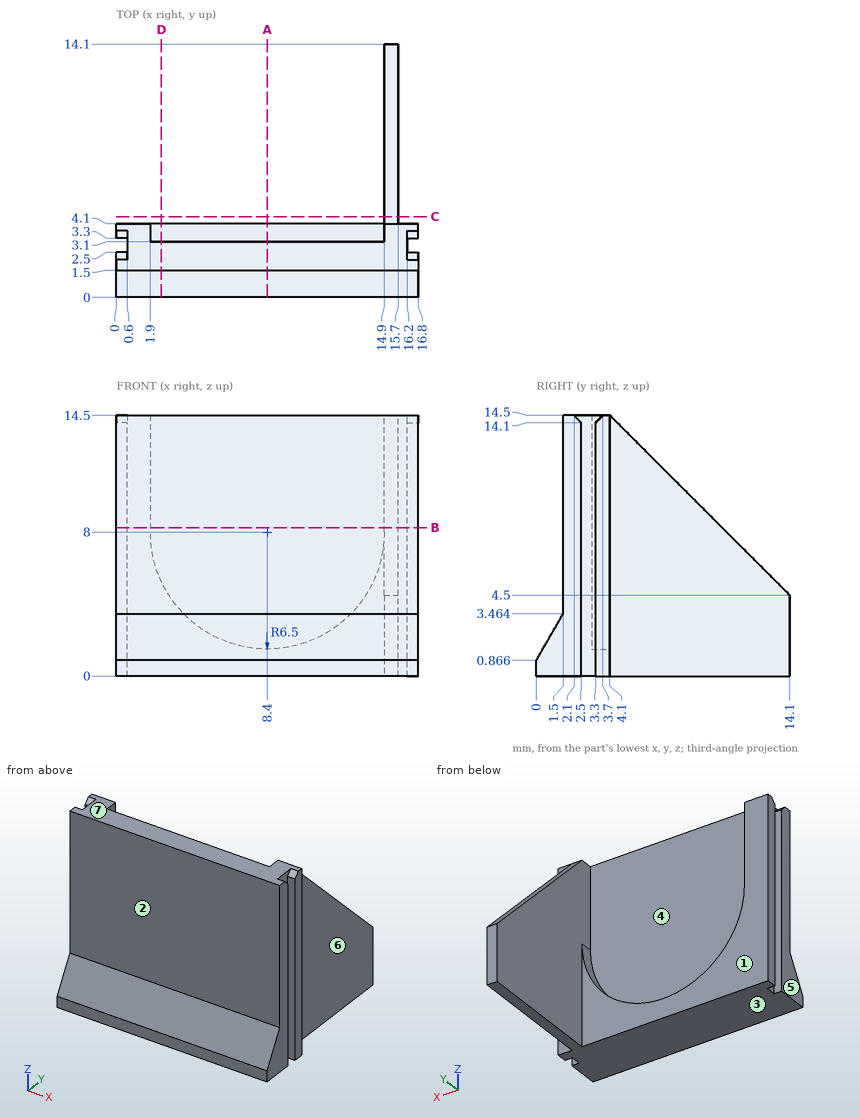
Answer from the drawing. Dimensions are ordinates in mm from the lowest x, y and z of the part. A direction names the side the tool comes from. Give positions to 0.01 mm unless a question says otherwise; leave off trailing zeros. Write each loop counter-clockwise with the first axis right and the second up, starting at its lowest first coordinate (ties: lowest second). Pieces come first, ordered by that corner, then holes. Notation, with made-up numbers: (68.5, 73.5) -> (109.5, 73.5) arc R32 ccw to (109.5, 99.5) -> close; hole circle Ø7 at (-12, 35.5). An arc over 180 degrees is marked (long way). Use a Markdown table: item, result.
(1) Section B-B, the plane z = 8.25 is taken. Determine the outline of the cut face in (x, y), then the cut area to 3 significant figures.
Return value:
| item | result |
|---|---|
| outline | (0, 1.5) -> (16.8, 1.5) -> (16.8, 2.5) -> (16.2, 2.5) -> (16.2, 3.3) -> (16.8, 3.3) -> (16.8, 4.1) -> (15.7, 4.1) -> (15.7, 10.35) -> (14.9, 10.35) -> (14.9, 3.1) -> (1.9, 3.1) -> (1.9, 4.1) -> (0, 4.1) -> (0, 3.3) -> (0.6, 3.3) -> (0.6, 2.5) -> (0, 2.5) -> close |
| area | 34.7 mm2 |
(2) Find the intervals of material crossed by probe 1 along Y at (x, z) = (3, 14.25); probe 2 along X at (y, z) = (8.25, 3.75); probe 3 along Y at (x, z) = (15.75, 13), in increasing order. Write a range as from..to.
Return value:
| item | result |
|---|---|
| probe 1 | 1.5..3.1 |
| probe 2 | 14.9..15.7 |
| probe 3 | 1.5..4.1 |
(3) For the marked faces 1, 2 and 3, determine the directions among +Z, -Z, +X, -X, +Y, -Y from which every point of the face is accessible in a straight line to the end or side of a thin tool.
Return value:
| item | result |
|---|---|
| face 1 | +Z, -Z, -X, +Y |
| face 2 | +Z, +X, -X, -Y |
| face 3 | -Z, +X, -X, +Y, -Y |
(4) Section A-A, the plane x = 8.4 is taken. Determine the outline of the cut face in (y, z).
Return value:
| item | result |
|---|---|
| outline | (0, 0) -> (4.1, 0) -> (4.1, 1.5) -> (3.1, 1.5) -> (3.1, 14.5) -> (1.5, 14.5) -> (1.5, 3.46) -> (0, 0.87) -> close |
(5) Section C-C, the plane y = 4.5 is taken. Determine the outline of the cut face in (x, z), then the cut area to 3 significant figures.
Return value:
| item | result |
|---|---|
| outline | (14.9, 0) -> (15.7, 0) -> (15.7, 14.1) -> (14.9, 14.1) -> close |
| area | 11.3 mm2 |
(6) Determine the mould class of the marked faces 4, 5, 6 and 7 for opening direction X: released by +X, released by -X, zero draft, split by the parting line, or undercut.
Return value:
| item | result |
|---|---|
| face 4 | undercut |
| face 5 | released by -X |
| face 6 | released by +X |
| face 7 | zero draft |
(7) Flat-ended cylindrical pins translate along their axes: P1, Ø0.7, axis at x = 16.5, z = 8.5, coming from the -Y side; P2, Ø1.2, axis at x = 16.5, z = 10, coming from the +Y side; P3, Ø3, axis at y = 7.5, z = 8.5, coming from the +X side. Find the tip coordinate at first contact, or state that the pin passes through.
Return value:
| item | result |
|---|---|
| P1 | y = 1.5 |
| P2 | y = 4.1 |
| P3 | x = 15.7 |
(8) Section D-D, the plane x = 2.5 is taken. Determine the outline of the cut face in (y, z), then the cut area to 3 significant figures.
Return value:
| item | result |
|---|---|
| outline | (0, 0) -> (4.1, 0) -> (4.1, 5.27) -> (3.1, 5.27) -> (3.1, 14.5) -> (1.5, 14.5) -> (1.5, 3.46) -> (0, 0.87) -> close |
| area | 31.7 mm2 |
